Work out the finished part from the listing and answer in its coordinate system (mm). Round coordinates to 2 decimals unless told otherwise and drop trailing zeros. Loops run counter-clockwise (first coordinate to the right, second up) from the corner with the lowest first, then second, coordinate; pieces in that order, holes last.
Autodesk Inventor part; units mm, degrees
ref_plane "YZ Plane" through (0, 0, 0) normal (1, 0, 0) x (0, 1, 0)
ref_plane "XZ Plane" through (0, 0, 0) normal (0, 1, 0) x (-1, 0, 0)
ref_plane "XY Plane" through (0, 0, 0) normal (0, 0, 1) x (1, 0, 0)
sketch "Sketch1" plane through (0, 0, 0) normal (0, 0, 1) x (1, 0, 0)
  line L0 (0, 0) -> (300.8, 0)
  line L1 (300.8, 0) -> (300.8, 250)
  line L2 (300.8, 250) -> (0, 250)
  line L3 (0, 250) -> (0, 0)
  dimension "d0" = 300.8
  dimension "d1" = 250
extrude "Extrusion1" add sketch "Sketch1" against normal blind 150
sketch "Sketch2" plane through (300.8, 0, 0) normal (1, 0, 0) x (0, 0, -1)
  line L0 (0, 0) -> (0, 250)
  line L1 (0, 250) -> (150, 250)
  point P0 (75, 200)
  point P1 (75, 50)
  dimension "d4" = 75
  dimension "d5" = 75
  dimension "d6" = 150
  dimension "d7" = 50
hole "Hole1" at (300.8, 200, -75) at (300.8, 50, -75) direction (-1, 0, 0) diameter 32 end through all
sketch "Sketch3" plane through (0, 0, 0) normal (0, 0, 1) x (1, 0, 0)
  line L0 (0, 0) -> (300.8, 0)
  line L1 (300.8, 250) -> (0, 250)
  line L2 (0, 250) -> (0, 0)
  line L3 (300.8, 0) -> (300.8, 250)
  point P0 (95.4, 125)
  point P1 (205.4, 125)
  dimension "d16" = 125
  dimension "d17" = 125
  dimension "d31" = 110
  dimension "d32" = 95.4
hole "Hole2" at (95.4, 125, 0) at (205.4, 125, 0) direction (0, 0, -1) diameter 26.4 end through all
chamfer "Chamfer1" distance 2 angle 45 2 edges at (150.4, 250, -150) (150.4, 250, 0)
properties part number "Soporte mesa"
1. Consider probe 1 along Y at (x, z) = (235, -75); probe 2 along X at (y, z) = (125, -83); probe 3 along Y at (x, z) = (205.4, -112). Determine where each line is inside the solid, lowest interval first.
Answer key:
probe 1: y = 0 to 34, 66 to 184, 216 to 250
probe 2: x = 0 to 82.2, 108.6 to 192.2, 218.6 to 300.8
probe 3: y = 0 to 111.8, 138.2 to 250
2. Find section A-A (x = 95.4). Write down the section's boundary in (y, z).
Answer key:
outline: (0, -150) - (111.8, -150) - (111.8, 0) - (0, 0) - close; (138.2, -150) - (248, -150) - (250, -148) - (250, -2) - (248, 0) - (138.2, 0) - close; hole circle Ø32 at (50, -75); hole circle Ø32 at (200, -75)
3. Find section B-B (z = -75). Write down the section's boundary in (x, y).
Answer key:
outline: (0, 0) - (300.8, 0) - (300.8, 34) - (0, 34) - close; (0, 66) - (300.8, 66) - (300.8, 184) - (0, 184) - close; (0, 216) - (300.8, 216) - (300.8, 250) - (0, 250) - close; hole circle Ø26.4 at (95.4, 125); hole circle Ø26.4 at (205.4, 125)
4. Determine the mould class of faces 1 (the face through (300.8, 123, -74)), 2 (the face through (148.294, 59.736, -62.303)), 3 (the face through (217.11, 118.91, -76.05)), 4 (the face through (153, 250, -74)) for opening direction Y: +Y half, -Y half, draft (parallel to the pull), parting line (faces both ways), or undercut.
Answer key:
face 1: draft
face 2: undercut
face 3: undercut
face 4: +Y half
5. Find section C-C (y = 50). Write down the section's boundary in (x, z), then the cut area to 3 significant figures.
Answer key:
outline: (0, -150) - (300.8, -150) - (300.8, -91) - (0, -91) - close; (0, -59) - (300.8, -59) - (300.8, 0) - (0, 0) - close
area: 35,500 mm2
6. Find section D-D (y = 125). Write down the section's boundary in (x, z).
Answer key:
outline: (0, -150) - (82.2, -150) - (82.2, 0) - (0, 0) - close; (108.6, -150) - (192.2, -150) - (192.2, 0) - (108.6, 0) - close; (218.6, -150) - (300.8, -150) - (300.8, 0) - (218.6, 0) - close
